The model under review builds one solid part; all positions refer to its coordinate system, in mm. Face numbers are marked on the shaded views. Coordinates: 2 decimals unless noted, no trailing zeros. Order: outer loops, then holes, each group sorted by start corner. A loop starts at its lowest first (then second) coordinate and runs counter-clockwise, first axis right, second up.
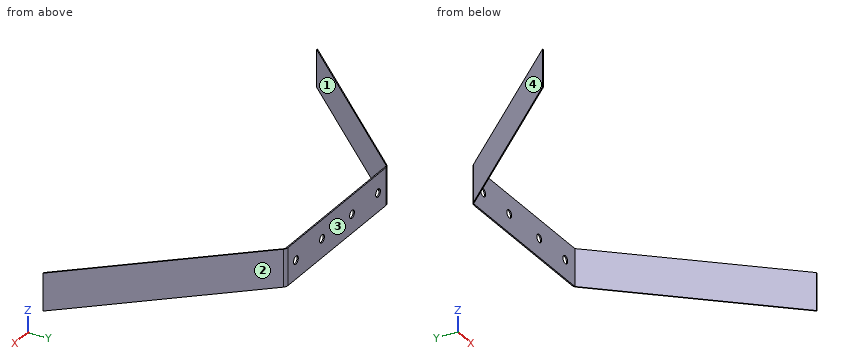
from build123d import *

# Parameters (mm, degrees)
SKETCH1_W           = 410
SKETCH1_H           = 195
BOSS_EXTRUDE1_DEPTH = 30
CUT_EXTRUDE1_DEPTH  = 30
CUT_EXTRUDE2_DEPTH  = 30
FILLET1_R           = 5
FILLET4_R           = 5
FILLET5_R           = 5
FILLET6_R           = 5
SKETCH4_R           = 1.65
CUT_EXTRUDE3_DEPTH  = 423.5
SKETCH5_R           = 3.175
CUT_EXTRUDE4_DEPTH  = 10
SKETCH7_W           = 30
SKETCH7_H           = 69
CUT_EXTRUDE6_DEPTH  = 420


with BuildPart() as part:
    # Sketch1 → Boss-Extrude1 (new body)
    with BuildSketch(Plane.XY):
        Rectangle(SKETCH1_W, SKETCH1_H)
    extrude(amount=BOSS_EXTRUDE1_DEPTH)

    # Sketch2 → Cut-Extrude1 (cut)
    with BuildSketch(Plane.XY.offset(30)):
        Polygon((-205, 97.5), (-205, -52.5), (-67.5, 97.5), align=None)
        Polygon((205, 97.5), (67.5, 97.5), (205, -52.5), align=None)
    extrude(amount=-CUT_EXTRUDE1_DEPTH, mode=Mode.SUBTRACT)

    # Sketch3 → Cut-Extrude2 (cut)
    with BuildSketch(Plane.XY.offset(30)):
        Polygon((-67.5, 96.5), (-204, -52.5), (-204, -97.5), (204, -97.5), (204, -52.5), (67.5, 96.5), align=None)
    extrude(amount=-CUT_EXTRUDE2_DEPTH, mode=Mode.SUBTRACT)

    # Fillet1
    fillet1_edges = [part.edges().sort_by_distance(p)[0] for p in [
        (-205, -52.5, 15),
    ]]
    fillet(fillet1_edges, radius=FILLET1_R)

    # Fillet4
    fillet4_edges = [part.edges().sort_by_distance(p)[0] for p in [
        (-67.5, 97.5, 15),
    ]]
    fillet(fillet4_edges, radius=FILLET4_R)

    # Fillet5
    fillet5_edges = [part.edges().sort_by_distance(p)[0] for p in [
        (67.5, 97.5, 15),
    ]]
    fillet(fillet5_edges, radius=FILLET5_R)

    # Fillet6
    fillet6_edges = [part.edges().sort_by_distance(p)[0] for p in [
        (205, -52.5, 15),
    ]]
    fillet(fillet6_edges, radius=FILLET6_R)

    # Sketch4 → Cut-Extrude3 (cut, through all)
    with BuildSketch(Plane(origin=(205, 0, 0), x_dir=(0, 0, -1), z_dir=(1, 0, 0))):
        with Locations(Location((-15, -75.972459226, 0), (0, 0, 90))):
            Circle(SKETCH4_R)
    extrude(amount=-CUT_EXTRUDE3_DEPTH, mode=Mode.SUBTRACT)

    # Sketch5 → Cut-Extrude4 (cut)
    with BuildSketch(Plane(origin=(0, 97.5, 0), x_dir=(1, 0, 0), z_dir=(0, 1, 0))):
        with Locations(Location((-20, -15, 0), (0, 0, 270))):
            Circle(SKETCH5_R)
        with Locations(Location((20, -15, 0), (0, 0, 270))):
            Circle(SKETCH5_R)
        with Locations(Location((54.768750122, -15, 0), (0, 0, 270))):
            Circle(SKETCH5_R)
        with Locations(Location((-54.768749878, -15, 0), (0, 0, 270))):
            Circle(SKETCH5_R)
    extrude(amount=-CUT_EXTRUDE4_DEPTH, mode=Mode.SUBTRACT)

    # Sketch7 → Cut-Extrude6 (cut)
    with BuildSketch(Plane(origin=(210, 0, 0), x_dir=(0, 0, -1), z_dir=(1, 0, 0))):
        with Locations((-15, -63)):
            Rectangle(SKETCH7_W, SKETCH7_H)
    extrude(amount=-CUT_EXTRUDE6_DEPTH, mode=Mode.SUBTRACT)


solid = part.part
(1) Consider section A-A (z = 15). Give the boundary of the cut face in (x, y) (1 decimal), then the cut area to 3 significant figures.
(2) Consider section D-D (x = -36). Give the boundary of the cut face in (y, z), then the cut area to 3 significant figures.
(3) The part is to be moulded in two halves that separate along X. For the marked faces 1, 2, 3 and 4, say which applies: +X half, -X half, draft (parallel to the pull), parting line (faces both ways), or undercut.
(4) Insertion check: pin 1 Ø3 at (x, z) = (-84, 16.5) entering from -Y; pin 2 Ø8.5 at (x, z) = (54.77, 15) entering from -Y; pin 3 Ø5.5 at (x, z) = (-54.77, 15) entering from +Y; pin 4 Ø1.5 at (x, z) = (-71.5, 25) entering from -Y (3 decimals). Each pin has a flat end and moves straight along its axis. Give the tip position at first contact, or say it passes through.
(5) Consider section C-C (y = 78). Give the boundary of the cut face in (x, z) (3 decimals), then the cut area to 3 significant figures.
(6) Wall thickness on line 1 (X direction, y = 97.1, z = 15) (3 decimals); line 2 (X direction, y = 96.85, z = 15) (3 decimals); line 3 (X direction, y = 74.5, z = 23.5): over which ranges is each line inside the solid? List them lowest first.
(7) Consider section B-B (x = 20). Give the boundary of the cut face in (y, z) (3 decimals), then the cut area to 4 significant figures.
Findings:
1. outline: (-183, -28.5) - (-182, -28.5) - (-67.5, 96.5) - (-57.9, 96.5) - (-57.9, 97.5) - (-65.3, 97.5) arc R5 ccw to (-69, 95.9) - close; (-51.6, 96.5) - (-23.2, 96.5) - (-23.2, 97.5) - (-51.6, 97.5) - close; (-16.8, 96.5) - (16.8, 96.5) - (16.8, 97.5) - (-16.8, 97.5) - close; (23.2, 96.5) - (51.6, 96.5) - (51.6, 97.5) - (23.2, 97.5) - close; (57.9, 96.5) - (67.5, 96.5) - (182, -28.5) - (183, -28.5) - (69, 95.9) arc R5 ccw to (65.3, 97.5) - (57.9, 97.5) - close
1. area: 347 mm2
2. outline: (96.5, 0) - (97.5, 0) - (97.5, 30) - (96.5, 30) - close
2. area: 30.0 mm2
3. face 1: undercut
3. face 2: +X half
3. face 3: draft
3. face 4: -X half
4. pin 1: stops at y = 76.85
4. pin 2: stops at y = 96.5
4. pin 3: passes through
4. pin 4: stops at y = 91.315
5. outline: (-85.375, 0) - (-84.448, 0) - (-84.448, 30) - (-85.375, 30) - close; (84.448, 0) - (85.375, 0) - (85.375, 30) - (84.448, 30) - close
5. area: 55.6 mm2
6. line 1: x = -67.26 to -57.944, -51.594 to -23.175, -16.825 to 16.825, 23.175 to 51.594, 57.944 to 67.26
6. line 2: x = -67.766 to -57.944, -51.594 to -23.175, -16.825 to 16.825, 23.175 to 51.594, 57.944 to 67.766
6. line 3: x = -88.58 to -87.65, 87.65 to 88.58
7. outline: (96.5, 0) - (97.5, 0) - (97.5, 11.825) - (96.5, 11.825) - close; (96.5, 18.175) - (97.5, 18.175) - (97.5, 30) - (96.5, 30) - close
7. area: 23.65 mm2
